Verification items for the finished model (mm, model axes). A direction names the side the tool comes from. Give positions to 0.01 mm unless a question says otherwise; leave off trailing zeros. Order: outer loops, then holes, each group sorted by start corner. A loop starts at its lowest first (then second) coordinate and runs counter-clockwise, first axis right, second up. Notation, with made-up numbers: (60.25, 65.25) - (92.25, 65.25) arc R22 cw to (92.25, 90.25) - close; hole circle Ø11 at (26.25, 27). An arc over 180 degrees is marked (long way). Answer as a JSON object with one key per item and string values. Group by question number.
(1) Depth check by flat-ended pin: pin 1 Ø4 at (y, z) = (12.5, 7) entering from +X; pin 2 Ø0.5 at (x, z) = (-15.5, 16.5) entering from +Y; pin 3 Ø3.5 at (x, z) = (33.5, -1.5) entering from +Y. Enter the tip coordinate at first touch or a pass-through.
(2) Section check A-A (z = -12.5). Record the boundary of the cut face in (x, y).
(3) Section check C-C (x = 24.5). Record the boundary of the cut face in (y, z), then the cut area to 3 significant figures.
(4) Thickness scan on line 1 (Y direction, x = 29.25, z = 0); line 2 (Y direction, x = 0, z = 14); line 3 (X direction, y = 37, z = 17). Record the ranges inside material, lowest first.
(5) Mould release check, pull along Y, two halves, no side actions. Record for faces 1 (the face through (0.42, 0.86, -21.6)), 2 (the face through (0, 9, -9.5)), 3 (the face through (33.57, 18.78, -21)): +Y half, -Y half, draft (parallel to the pull), parting line (faces both ways), or undercut.
(6) Section check B-B (x = 15.25). Record the boundary of the cut face in (y, z).
(7) Access from +Z, -Z, +X, -X, +Y, -Y to the whole of each face (thin tool, end or side, straight path). Record for faces 4 (the face through (10, 15, 21)), 5 (the face through (-34, 15, -10)), 6 (the face through (33.521, 23.859, 8.797)), 7 (the face through (0, 25, -21)), 8 (the face through (-15, 34, -16)).
(8) Section check D-D (x = -18). Record the boundary of the cut face in (y, z), then the cut area to 3 significant figures.
```python
from build123d import *

# Parameters (mm, degrees)
SKETCH1_W           = 70
SKETCH1_H           = 45
BOSS_EXTRUDE1_DEPTH = 40
SKETCH2_R           = 2
CUT_EXTRUDE1_DEPTH  = 10
CUT_EXTRUDE2_DEPTH  = 3
SKETCH4_R           = 2
CUT_EXTRUDE3_DEPTH  = 10
CUT_EXTRUDE4_DEPTH  = 3
SKETCH8_R           = 2
CUT_EXTRUDE5_DEPTH  = 10
FILLET1_R           = 3
FILLET2_R           = 5
SKETCH9_W           = 31
SKETCH9_H           = 7
CUT_EXTRUDE6_DEPTH  = 55
SKETCH10_R          = 2
CUT_EXTRUDE7_DEPTH  = 6
SKETCH11_R          = 7.5
CUT_EXTRUDE8_DEPTH  = 14
FILLET3_R           = 5


with BuildPart() as part:
    # Sketch1 → Boss-Extrude1 (new body)
    with BuildSketch(Plane(origin=(0, 0, 0), x_dir=(1, 0, 0), z_dir=(0, 1, 0))):
        Rectangle(SKETCH1_W, SKETCH1_H)
    extrude(amount=BOSS_EXTRUDE1_DEPTH)

    # Sketch2 → Cut-Extrude1 (cut)
    with BuildSketch(Plane.XZ):
        with Locations(Location((-28, 15.5, 0), (0, 0, 270))):
            Circle(SKETCH2_R)
        with Locations(Location((28, 15.5, 0), (0, 0, 90))):
            Circle(SKETCH2_R)
        with Locations(Location((28, -16.330849274, 0), (0, 0, 270))):
            Circle(SKETCH2_R)
        with Locations(Location((-28, -16.330849274, 0), (0, 0, 90))):
            Circle(SKETCH2_R)
    extrude(amount=-CUT_EXTRUDE1_DEPTH, mode=Mode.SUBTRACT)

    # Sketch3 → Cut-Extrude2 (cut)
    with BuildSketch(Plane(origin=(35, 0, 0), x_dir=(0, 0, -1), z_dir=(1, 0, 0))):
        with BuildLine():
            Line((-6, 5), (6, 5))
            ThreePointArc((6, 5), (8.828427125, 6.171572875), (10, 9))
            Line((10, 9), (10, 21))
            ThreePointArc((10, 21), (8.828427125, 23.828427125), (6, 25))
            Line((6, 25), (-6, 25))
            ThreePointArc((-6, 25), (-8.828427125, 23.828427125), (-10, 21))
            Line((-10, 21), (-10, 9))
            ThreePointArc((-10, 9), (-8.828427125, 6.171572875), (-6, 5))
        make_face()
    cut_extrude2 = extrude(amount=-CUT_EXTRUDE2_DEPTH, mode=Mode.SUBTRACT)

    # Sketch4 → Cut-Extrude3 (cut)
    with BuildSketch(Plane(origin=(32, 0, 0), x_dir=(0, 0, -1), z_dir=(1, 0, 0))):
        with Locations((0, 21)):
            Circle(SKETCH4_R)
        with Locations((0, 9)):
            Circle(SKETCH4_R)
    cut_extrude3 = extrude(amount=-CUT_EXTRUDE3_DEPTH, mode=Mode.SUBTRACT)

    # Mirror1: Cut-Extrude2, Cut-Extrude3 across plane
    add(cut_extrude2.mirror(Plane(origin=(0, 0, 0), x_dir=(0, 0, 1), z_dir=(1, 0, 0))), mode=Mode.SUBTRACT)
    add(cut_extrude3.mirror(Plane(origin=(0, 0, 0), x_dir=(0, 0, 1), z_dir=(1, 0, 0))), mode=Mode.SUBTRACT)

    # Sketch7 → Cut-Extrude4 (cut)
    with BuildSketch(Plane(origin=(0, 0, -22.5), x_dir=(-1, 0, 0), z_dir=(0, 0, -1))):
        with BuildLine():
            Line((-6, 5), (6, 5))
            ThreePointArc((6, 5), (8.828427125, 6.171572875), (10, 9))
            Line((10, 9), (10, 21))
            ThreePointArc((10, 21), (8.828427125, 23.828427125), (6, 25))
            Line((6, 25), (-6, 25))
            ThreePointArc((-6, 25), (-8.828427125, 23.828427125), (-10, 21))
            Line((-10, 21), (-10, 9))
            ThreePointArc((-10, 9), (-8.828427125, 6.171572875), (-6, 5))
        make_face()
    cut_extrude4 = extrude(amount=-CUT_EXTRUDE4_DEPTH, mode=Mode.SUBTRACT)

    # Sketch8 → Cut-Extrude5 (cut)
    with BuildSketch(Plane(origin=(0, 0, -19.5), x_dir=(-1, 0, 0), z_dir=(0, 0, -1))):
        with Locations((0, 21)):
            Circle(SKETCH8_R)
        with Locations((0, 9)):
            Circle(SKETCH8_R)
    cut_extrude5 = extrude(amount=-CUT_EXTRUDE5_DEPTH, mode=Mode.SUBTRACT)

    # Mirror2: Cut-Extrude4, Cut-Extrude5 across plane
    add(cut_extrude4.mirror(Plane.XY), mode=Mode.SUBTRACT)
    add(cut_extrude5.mirror(Plane.XY), mode=Mode.SUBTRACT)

    # Fillet1
    fillet1_edges = [part.edges().sort_by_distance(p)[0] for p in [
        (-35, 0, 0),
        (0, 0, -22.5),
        (35, 0, 0),
        (0, 0, 22.5),
    ]]
    fillet(fillet1_edges, radius=FILLET1_R)

    # Fillet2
    # the kernel refuses this fillet: 5 mm, written as the material it takes off along each edge
    with BuildSketch(Plane(origin=(-30, 0, 17.5), x_dir=(0, 0, 1), z_dir=(1, 0, 0))) as fillet2_piece_1:
        with BuildLine():
            CenterArc((2, -3), 3, 0, 90)
            Line((5, -3), (5, 0))
            Line((5, 0), (2, 0))
        make_face()
    revolve(axis=Axis((-30, 0, 17.5), (0, -1, 0)), revolution_arc=90, mode=Mode.SUBTRACT)
    with BuildSketch(Plane(origin=(-30, 0, -17.5), x_dir=(-1, 0, 0), z_dir=(0, 0, 1))) as fillet2_piece_2:
        with BuildLine():
            CenterArc((2, -3), 3, 0, 90)
            Line((5, -3), (5, 0))
            Line((5, 0), (2, 0))
        make_face()
    revolve(axis=Axis((-30, 0, -17.5), (0, -1, 0)), revolution_arc=90, mode=Mode.SUBTRACT)
    with BuildSketch(Plane(origin=(30, 0, 17.5), x_dir=(1, 0, 0), z_dir=(0, 0, -1))) as fillet2_piece_3:
        with BuildLine():
            CenterArc((2, -3), 3, 0, 90)
            Line((5, -3), (5, 0))
            Line((5, 0), (2, 0))
        make_face()
    revolve(axis=Axis((30, 0, 17.5), (0, -1, 0)), revolution_arc=90, mode=Mode.SUBTRACT)
    with BuildSketch(Plane(origin=(30, 0, -17.5), x_dir=(0, 0, -1), z_dir=(-1, 0, 0))) as fillet2_piece_4:
        with BuildLine():
            CenterArc((2, -3), 3, 0, 90)
            Line((5, -3), (5, 0))
            Line((5, 0), (2, 0))
        make_face()
    revolve(axis=Axis((30, 0, -17.5), (0, -1, 0)), revolution_arc=90, mode=Mode.SUBTRACT)
    with BuildSketch(Plane(origin=(-35, 0, 22.5), x_dir=(1, 0, 0), z_dir=(0, 1, 0)), Plane(origin=(-35, 0, -22.5), x_dir=(0, 0, 1), z_dir=(0, 1, 0))) as fillet2_piece_5:
        with BuildLine():
            CenterArc((FILLET2_R, FILLET2_R), FILLET2_R, 180, 90)
            Line((0, FILLET2_R), (0, 0))
            Line((0, 0), (FILLET2_R, 0))
        make_face()
    extrude(amount=52.5, mode=Mode.SUBTRACT)
    with BuildSketch(Plane(origin=(35, 0, -22.5), x_dir=(0, 0, 1), z_dir=(0, 1, 0)), Plane(origin=(35, 0, 22.5), x_dir=(-1, 0, 0), z_dir=(0, 1, 0))) as fillet2_piece_6:
        with BuildLine():
            CenterArc((FILLET2_R, -FILLET2_R), FILLET2_R, 90, 90)
            Line((0, -FILLET2_R), (0, 0))
            Line((0, 0), (FILLET2_R, 0))
        make_face()
    extrude(amount=52.5, mode=Mode.SUBTRACT)

    # Sketch9 → Cut-Extrude6 (cut)
    with BuildSketch(Plane.ZY.offset(35)):
        with Locations((0, 32)):
            Rectangle(SKETCH9_W, SKETCH9_H)
    extrude(amount=-CUT_EXTRUDE6_DEPTH, mode=Mode.SUBTRACT)

    # Sketch10 → Cut-Extrude7 (cut)
    with BuildSketch(Plane(origin=(0, 40, 0), x_dir=(1, 0, 0), z_dir=(0, 1, 0))):
        with Locations(Location((15.25, 15.25, 0), (0, 0, 270))):
            Circle(SKETCH10_R)
        with Locations(Location((15.25, -15.25, 0), (0, 0, 270))):
            Circle(SKETCH10_R)
        with Locations(Location((-15.25, 15.25, 0), (0, 0, 270))):
            Circle(SKETCH10_R)
        with Locations(Location((-15.25, -15.25, 0), (0, 0, 270))):
            Circle(SKETCH10_R)
    extrude(amount=-CUT_EXTRUDE7_DEPTH, mode=Mode.SUBTRACT)

    # Sketch11 → Cut-Extrude8 (cut)
    with BuildSketch(Plane(origin=(35, 0, 0), x_dir=(0, 0, -1), z_dir=(1, 0, 0))):
        with Locations((0, 40)):
            Circle(SKETCH11_R)
    extrude(amount=-CUT_EXTRUDE8_DEPTH, mode=Mode.SUBTRACT)

    # Fillet3
    # the kernel refuses this fillet: 5 mm, written as the material it takes off along each edge
    with BuildSketch(Plane(origin=(35, 40, 5), x_dir=(-1, 0, 0), z_dir=(0, 0, -1)), Plane(origin=(35, 40, 17.5), x_dir=(-1, 0, 0), z_dir=(0, 0, -1))) as fillet3_piece_1:
        with BuildLine():
            CenterArc((FILLET3_R, -FILLET3_R), FILLET3_R, 90, 90)
            Line((0, -FILLET3_R), (0, 0))
            Line((0, 0), (FILLET3_R, 0))
        make_face()
    extrude(amount=22.5, mode=Mode.SUBTRACT)
    with BuildSketch(Plane(origin=(30, 40, -17.5), x_dir=(0, 0, -1), z_dir=(-1, 0, 0))) as fillet3_piece_2:
        with BuildLine():
            CenterArc((5 - FILLET3_R, FILLET3_R), FILLET3_R, 270, 90)
            Line((5, FILLET3_R), (5, 0))
            Line((5, 0), (5 - FILLET3_R, 0))
        make_face()
    revolve(axis=Axis((30, 40, -17.5), (0, -1, 0)), revolution_arc=90, mode=Mode.SUBTRACT)
    with BuildSketch(Plane(origin=(30, 40, -22.5), x_dir=(0, 0, 1), z_dir=(-1, 0, 0))) as fillet3_piece_3:
        with BuildLine():
            CenterArc((FILLET3_R, -FILLET3_R), FILLET3_R, 90, 90)
            Line((0, -FILLET3_R), (0, 0))
            Line((0, 0), (FILLET3_R, 0))
        make_face()
    extrude(amount=60, mode=Mode.SUBTRACT)
    with BuildSketch(Plane(origin=(-30, 40, -17.5), x_dir=(-1, 0, 0), z_dir=(0, 0, 1))) as fillet3_piece_4:
        with BuildLine():
            CenterArc((5 - FILLET3_R, FILLET3_R), FILLET3_R, 270, 90)
            Line((5, FILLET3_R), (5, 0))
            Line((5, 0), (5 - FILLET3_R, 0))
        make_face()
    revolve(axis=Axis((-30, 40, -17.5), (0, -1, 0)), revolution_arc=90, mode=Mode.SUBTRACT)
    with BuildSketch(Plane(origin=(-35, 40, -17.5), x_dir=(1, 0, 0), z_dir=(0, 0, 1))) as fillet3_piece_5:
        with BuildLine():
            CenterArc((FILLET3_R, -FILLET3_R), FILLET3_R, 90, 90)
            Line((0, -FILLET3_R), (0, 0))
            Line((0, 0), (FILLET3_R, 0))
        make_face()
    extrude(amount=35, mode=Mode.SUBTRACT)
    with BuildSketch(Plane(origin=(-30, 40, 17.5), x_dir=(0, 0, 1), z_dir=(1, 0, 0))) as fillet3_piece_6:
        with BuildLine():
            CenterArc((5 - FILLET3_R, FILLET3_R), FILLET3_R, 270, 90)
            Line((5, FILLET3_R), (5, 0))
            Line((5, 0), (5 - FILLET3_R, 0))
        make_face()
    revolve(axis=Axis((-30, 40, 17.5), (0, -1, 0)), revolution_arc=90, mode=Mode.SUBTRACT)
    with BuildSketch(Plane(origin=(30, 40, 17.5), x_dir=(1, 0, 0), z_dir=(0, 0, -1))) as fillet3_piece_7:
        with BuildLine():
            CenterArc((5 - FILLET3_R, FILLET3_R), FILLET3_R, 270, 90)
            Line((5 - FILLET3_R, 0), (5, 0))
            Line((5, 0), (5, FILLET3_R))
        make_face()
    revolve(axis=Axis((30, 40, 17.5), (0, -1, 0)), revolution_arc=90, mode=Mode.SUBTRACT)
    with BuildSketch(Plane(origin=(-30, 40, 22.5), x_dir=(0, -1, 0), z_dir=(1, 0, 0))) as fillet3_piece_8:
        with BuildLine():
            CenterArc((FILLET3_R, FILLET3_R), FILLET3_R, 180, 90)
            Line((0, FILLET3_R), (0, 0))
            Line((0, 0), (FILLET3_R, 0))
        make_face()
    extrude(amount=60, mode=Mode.SUBTRACT)


solid = part.part
```
Solutions:
{
 "1": {"pin 1": "stops at x = 32", "pin 2": "stops at y = 34", "pin 3": "stops at y = 33.24"},
 "2": {"outline": "(-35, 3) arc R3 ccw to (-32, 0) - (32, 0) arc R3 ccw to (35, 3) - (35, 35) arc R5 ccw to (30, 40) - (-30, 40) arc R5 ccw to (-34.97, 35.5) - (20, 35.5) - (20, 28.5) - (-35, 28.5) - close; hole circle Ø4 at (0, 9); hole circle Ø4 at (0, 21)"},
 "3": {"outline": "(0, -19.5) arc R3 ccw to (3, -22.5) - (35, -22.5) arc R5 ccw to (40, -17.5) - (40, -7.5) arc R7.5 cw to (40, 7.5) - (40, 17.5) arc R5 ccw to (35, 22.5) - (3, 22.5) arc R3 ccw to (0, 19.5) - close; hole circle Ø4 at (9, 0); hole circle Ø4 at (21, 0)", "area": "1,670 mm2"},
 "4": {"line 1": "y = 0 to 7, 11 to 19, 23 to 32.5", "line 2": "y = 0 to 7, 11 to 19, 23 to 28.5, 35.5 to 40", "line 3": "x = -34.58 to -16.22, -14.28 to 14.28, 16.22 to 34.58"},
 "5": {"face 1": "-Y half", "face 2": "undercut", "face 3": "draft"},
 "6": {"outline": "(0, -19.5) arc R3 ccw to (3, -22.5) - (35, -22.5) arc R5 ccw to (40, -17.5) - (40, -17.25) - (34, -17.25) - (34, -15.5) - (28.5, -15.5) - (28.5, 15.5) - (34, 15.5) - (34, 17.25) - (40, 17.25) - (40, 17.5) arc R5 ccw to (35, 22.5) - (3, 22.5) arc R3 ccw to (0, 19.5) - close; (35.5, -13.25) - (40, -13.25) - (40, 13.25) - (35.5, 13.25) - close"},
 "7": {"face 4": "+Z", "face 5": "-X", "face 6": "+X", "face 7": "-Z", "face 8": "+Y"},
 "8": {"outline": "(0, -19.5) arc R3 ccw to (3, -22.5) - (35, -22.5) arc R5 ccw to (40, -17.5) - (40, 17.5) arc R5 ccw to (35, 22.5) - (3, 22.5) arc R3 ccw to (0, 19.5) - close; hole (28.5, -15.5) - (35.5, -15.5) - (35.5, 15.5) - (28.5, 15.5) - close", "area": "1,570 mm2"}
}
